```python
from build123d import *

# Parameters (mm, degrees)
BOSS_EXTRUDE1_DEPTH      = 8
FILLET1_R                = 2.5
BOSS_EXTRUDE2_DEPTH      = 9
BOSS_EXTRUDE2_DEPTH_BACK = 1
FILLET2_R                = 0.5
BOSS_EXTRUDE3_DEPTH      = 2.5
BOSS_EXTRUDE3_DEPTH_BACK = 1
SKETCH4_R                = 1.25
CUT_EXTRUDE1_DEPTH       = 9
CUT_EXTRUDE2_DEPTH       = 4
BOSS_EXTRUDE4_DEPTH      = 1
BOSS_EXTRUDE4_DEPTH_BACK = 1
SKETCH6_R                = 3
SKETCH7_R                = 1.25
CUT_EXTRUDE3_DEPTH       = 5


with BuildPart() as part:
    # Sketch1 → Boss-Extrude1 (new body)
    with BuildSketch(Plane(origin=(0, 0, 0), x_dir=(1, 0, 0), z_dir=(0, 1, 0))):
        with BuildLine():
            Line((-20, 3.5), (20, 3.5))
            ThreePointArc((20, 3.5), (23.5, 0), (20, -3.5))
            Line((20, -3.5), (-20, -3.5))
            ThreePointArc((-20, -3.5), (-23.5, 0), (-20, 3.5))
        make_face()
    extrude(amount=BOSS_EXTRUDE1_DEPTH)

    # Fillet1
    fillet1_edges = [part.edges().sort_by_distance(p)[0] for p in [
        (23.5, 8, 0),
        (0, 8, -3.5),
        (-23.5, 8, 0),
        (0, 8, 3.5),
    ]]
    fillet(fillet1_edges, radius=FILLET1_R)

    # Sketch2 → Boss-Extrude2 (add, two sides: drawn at the far end of the back side and taken through both)
    with BuildSketch(Plane(origin=(0, 8, 0), x_dir=(1, 0, 0), z_dir=(0, 1, 0)).offset(-BOSS_EXTRUDE2_DEPTH_BACK)):
        with BuildLine():
            Line((-12.5, 1.5), (12.5, 1.5))
            ThreePointArc((12.5, 1.5), (14, 0), (12.5, -1.5))
            Line((12.5, -1.5), (-12.5, -1.5))
            ThreePointArc((-12.5, -1.5), (-14, 0), (-12.5, 1.5))
        make_face()
    extrude(amount=BOSS_EXTRUDE2_DEPTH + BOSS_EXTRUDE2_DEPTH_BACK)

    # Fillet2
    fillet2_edges = [part.edges().sort_by_distance(p)[0] for p in [
        (-14, 17, 0),
        (0, 17, 1.5),
        (14, 17, 0),
        (0, 17, -1.5),
    ]]
    fillet(fillet2_edges, radius=FILLET2_R)

    # Sketch3 → Boss-Extrude3 (add, two sides: drawn at the far end of the back side and taken through both)
    with BuildSketch(Plane(origin=(0, 8, 0), x_dir=(1, 0, 0), z_dir=(0, 1, 0)).offset(-BOSS_EXTRUDE3_DEPTH_BACK)):
        with BuildLine():
            Line((-17.319048676, 0.75), (-13.799038106, 0.75))
            ThreePointArc((-13.799038106, 0.75), (-14, 0), (-13.799038106, -0.75))
            Line((-13.799038106, -0.75), (-17.319048676, -0.75))
            ThreePointArc((-17.319048676, -0.75), (-17.952914367, -0.890509549), (-18.468027815, -1.285714286))
            ThreePointArc((-18.468027815, -1.285714286), (-22, 0), (-18.468027815, 1.285714286))
            ThreePointArc((-18.468027815, 1.285714286), (-17.952914367, 0.890509549), (-17.319048676, 0.75))
        make_face()
        with BuildLine():
            Line((17.319048676, -0.75), (13.799038106, -0.75))
            ThreePointArc((13.799038106, -0.75), (14, 0), (13.799038106, 0.75))
            Line((13.799038106, 0.75), (17.319048676, 0.75))
            ThreePointArc((17.319048676, 0.75), (17.952914367, 0.890509549), (18.468027815, 1.285714286))
            ThreePointArc((18.468027815, 1.285714286), (22, 0), (18.468027815, -1.285714286))
            ThreePointArc((18.468027815, -1.285714286), (17.952914367, -0.890509549), (17.319048676, -0.75))
        make_face()
    extrude(amount=BOSS_EXTRUDE3_DEPTH + BOSS_EXTRUDE3_DEPTH_BACK)

    # Sketch4 → Cut-Extrude1 (cut)
    with BuildSketch(Plane.XZ):
        with Locations(Location((20, 0, 0), (0, 0, 270))):
            Circle(SKETCH4_R)
        with Locations(Location((-20, 0, 0), (0, 0, 270))):
            Circle(SKETCH4_R)
    extrude(amount=-CUT_EXTRUDE1_DEPTH, mode=Mode.SUBTRACT)

    # Sketch5 → Cut-Extrude2 (cut)
    with BuildSketch(Plane.XZ):
        with BuildLine():
            Line((8.51994599, 1.25), (-8.51994599, 1.25))
            ThreePointArc((-8.51994599, 1.25), (-11.157492475, 0.157492475), (-12.25, -2.48005401))
            Line((-12.25, -2.48005401), (-12.25, -3.5))
            Line((-12.25, -3.5), (12.25, -3.5))
            Line((12.25, -3.5), (12.25, -2.48005401))
            ThreePointArc((12.25, -2.48005401), (11.157492475, 0.157492475), (8.51994599, 1.25))
        make_face()
    extrude(amount=-CUT_EXTRUDE2_DEPTH, mode=Mode.SUBTRACT)

    # Sketch6 → Boss-Extrude4 (add, two sides: drawn at the far end of the back side and taken through both)
    with BuildSketch(Plane(origin=(0, 0, -3.5), x_dir=(-1, 0, 0), z_dir=(0, 0, -1)).offset(-BOSS_EXTRUDE4_DEPTH_BACK)):
        with Locations((-16.25, 3.79375)):
            Circle(SKETCH6_R)
        with Locations(Location((16.25, 3.79375, 0), (0, 0, 34.663105373))):
            Circle(SKETCH6_R)
    extrude(amount=BOSS_EXTRUDE4_DEPTH + BOSS_EXTRUDE4_DEPTH_BACK)

    # Sketch7 → Cut-Extrude3 (cut)
    with BuildSketch(Plane(origin=(0, 0, -4.5), x_dir=(-1, 0, 0), z_dir=(0, 0, -1))):
        with Locations((-16.25, 3.79375)):
            Circle(SKETCH7_R)
        with Locations((16.25, 3.79375)):
            Circle(SKETCH7_R)
    extrude(amount=-CUT_EXTRUDE3_DEPTH, mode=Mode.SUBTRACT)


solid = part.part
```
For this review, take the finished solid that the model builds, in its own axes (mm). A direction names the side the tool comes from. Round coordinates to 2 decimals unless told otherwise and drop trailing zeros. Write each loop counter-clockwise with the first axis right and the second up, starting at its lowest first coordinate (ties: lowest second). Pieces come first, ordered by that corner, then holes. Notation, with made-up numbers: (80, 53) -> (87, 53) arc R27 ccw to (87, 73) -> close; hole circle Ø8 at (77.5, -24.75). An arc over 180 degrees is marked (long way). One line per question, with ' | ' between items. Start each with the question number.
1) Add section A-A (y = 8.5). Write out the cut boundary in (x, z).
2) Add section B-B (x = 16.25). Write out the cut boundary in (y, z).
3) Mouldability with a two-part tool opening along Y and no side actions: class faces 1 (the flat face through (-12.25, 2, -3)), 2 (the flat face through (-16, 4, 0.5)), 3 (the flat face through (-19, 10.5, 0)) as +Y half, -Y half, draft (parallel to the pull), parting line (faces both ways), or undercut.
4) Add section C-C (z = -4). Write out the cut boundary in (x, y).
5) Machinability: for faces 4 (the cylindrical face through (17.17, 4.64, -2.04)), 5 (the flat face through (0, 4, -1)), 6 (the cylindrical face through (22, 9, 0)), 7 (the cylindrical face through (18.78, 4.44, 0.27)), 8 (the cylindrical face through (17.945, 9.224, -0.887)), which of the approach directions +Z, -Z, +X, -X, +Y, -Y give a long, thin tool a straight path to every point of the face, cutting with its end or side? Answer none if there is none.
6) For pin 1 Ø3 at (x, y) = (16, 8.5) entering from -Z; pin 2 Ø1.2 at (x, y) = (-1.5, 2.5) entering from -Z; pin 3 Ø9.5 at (x, y) = (2, 12.5) entering from +Z, all flat-tipped, find the tip position at first contact; note any pin that passes through.
7) Add section D-D (z = -0.25). Count the separate pieces of the cut face and the enclosed holes in it, and give its area (3 significant figures).
8) Wall thickness on line 1 along Y through (x, z) = (-16.25, -0.8); line 2 along X through (y, z) = (5.25, 0); line 3 along Y through (x, z) = (-16.25, -2): over which ranges is each line inside the solid? List them lowest first.
Reported:
1) outline: (-18.47, -1.29) arc R1.5 cw to (-17.32, -0.75) -> (-13.8, -0.75) arc R1.5 ccw to (-12.5, -1.5) -> (12.5, -1.5) arc R1.5 ccw to (13.8, -0.75) -> (17.32, -0.75) arc R1.5 cw to (18.47, -1.29) arc R2 ccw (long way) to (18.47, 1.29) arc R1.5 cw to (17.32, 0.75) -> (13.8, 0.75) arc R1.5 ccw to (12.5, 1.5) -> (-12.5, 1.5) arc R1.5 ccw to (-13.8, 0.75) -> (-17.32, 0.75) arc R1.5 cw to (-18.47, 1.29) arc R2 ccw (long way) to start; hole circle Ø2.5 at (-20, 0); hole circle Ø2.5 at (20, 0)
2) outline: (0, -3.5) -> (0.79, -3.5) -> (0.79, -4.5) -> (2.54, -4.5) -> (2.54, 0.5) -> (5.04, 0.5) -> (5.04, -4.5) -> (6.79, -4.5) -> (6.79, -3.14) arc R2.5 ccw to (8, -1) -> (8, -0.75) -> (10.5, -0.75) -> (10.5, 0.75) -> (8, 0.75) -> (8, 1) arc R2.5 ccw to (5.5, 3.5) -> (0, 3.5) -> close
3) face 1: draft | face 2: undercut | face 3: +Y half
4) outline: circle Ø6 at (-16.25, 3.79); circle Ø6 at (16.25, 3.79); hole circle Ø2.5 at (-16.25, 3.79); hole circle Ø2.5 at (16.25, 3.79)
5) face 4: -Z | face 5: -Z, -Y | face 6: +Y | face 7: -Y | face 8: -Z, +Y
6) pin 1: stops at z = -3 | pin 2: stops at z = 1.25 | pin 3: stops at z = 2.09
7) separate pieces: 1 | enclosed holes: 2 | area: 519 mm²
8) line 1: y = 0 to 2.54, 5.04 to 8 | line 2: x = -23.5 to -21.25, -18.75 to 18.75, 21.25 to 23.5 | line 3: y = 0 to 2.54, 5.04 to 7.79
